```python
from build123d import *

# Parameters (mm, degrees)
F0_R     = 7.5
F1_DEPTH = 2
F2_R     = 4
F3_DEPTH = 2.25
F4_R     = 2.2
F5_DEPTH = 4.251
F6_R     = 0.5


with BuildPart() as f1:
    # F0 (on Front) → F1 (new body)
    with BuildSketch(Plane.XZ):
        Circle(F0_R)
    extrude(amount=F1_DEPTH)

    # F2 (on face) → F3 (join)
    with BuildSketch(Plane.XZ.offset(2)):
        Circle(F2_R)
    extrude(amount=F3_DEPTH)

    # F4 (on face) → F5 (cut, through all)
    with BuildSketch(Plane.XZ.offset(4.25)):
        Circle(F4_R)
    extrude(amount=-F5_DEPTH, mode=Mode.SUBTRACT)

    # F6
    f6_edges = [f1.edges().sort_by_distance(p)[0] for p in [
        (-7.5, 0, 0),
    ]]
    fillet(f6_edges, radius=F6_R)


solid = f1.part
```
Can you work these out from the model? Positions are in its coordinate system, mm. A direction names the side the tool comes from. Give positions to 0.01 mm unless a question says otherwise; leave off trailing zeros. Order: outer loops, then holes, each group sorted by start corner. A loop starts at its lowest first (then second) coordinate and runs counter-clockwise, first axis right, second up. Notation, with made-up numbers: (23, 37) - (60, 37) arc R21 ccw to (60, 62) - close; hole circle Ø9 at (50.5, -8.75). An arc over 180 degrees is marked (long way). Use a Markdown table: item, result. Add a question column.
Q1. On a 3-axis mill with a long thin cutter (end or side, diameter ignored), from which of +Z, -Z, +X, -X, +Y, -Y can I reach the whole of each face in a straight line? I mean faces 4 (the flat face through (-2, 0, 2)), 5 (the flat face through (3, -2, -3)). Say none if no direction works.
Q2. If we section it at B-B on x = 0: Write out the boundary of the cut face in (y, z).
Q3. I'm going to push a flat-ended pin straight in: pin 1 (2 mm diameter, centred on x = -2, y = -2, fed in from -Z). Where does the tip first touch, or does it pass through?
Q4. If we section it at D-D on y = -3.35: Write out the boundary of the cut face in (x, z).
Q5. If we section it at C-C on y = -1.6: Write out the boundary of the cut face in (x, z).
Q6. If we mould it in two halves opening along Z, with no side actions, what happens to faces 1 (the cylindrical face through (-7.493, -1.24, 0.33)), 2 (the cylindrical face through (2.1, -2.15, 0.66)), 3 (the flat face through (2, -4.25, -2))? For each: released by +Z, released by -Z, zero draft, split by the parting line, or undercut.
Q7. Please list where these lines run through material, in increasing order: line 1 along Z through (x, y) = (0, -2.9); line 2 along Y through (x, z) = (-5.5, -2.5); line 3 along X through (y, z) = (-2.8, 1.75).
Q8. If we section it at A-A on z = 0: Write out the boundary of the cut face in (x, y), plus the area to 3 significant figures.
Answers follow:
| question | item | result |
|---|---|---|
| 1 | face 4 | +Z, -Z, +X, -X, +Y |
| 1 | face 5 | -Y |
| 2 | outline | (-4.25, -4) - (-2, -4) - (-2, -7.5) - (-0.5, -7.5) arc R0.5 ccw to (0, -7) - (0, -2.2) - (-4.25, -2.2) - close; (-4.25, 2.2) - (0, 2.2) - (0, 7) arc R0.5 ccw to (-0.5, 7.5) - (-2, 7.5) - (-2, 4) - (-4.25, 4) - close |
| 3 | pin 1 | stops at z = -7.43 |
| 4 | outline | circle Ø8 at (0, 0); hole circle Ø4.4 at (0, 0) |
| 5 | outline | circle Ø15 at (0, 0); hole circle Ø4.4 at (0, 0) |
| 6 | face 1 | split by the parting line |
| 6 | face 2 | undercut |
| 6 | face 3 | zero draft |
| 7 | line 1 | z = -4 to -2.2, 2.2 to 4 |
| 7 | line 2 | y = -2 to 0 |
| 7 | line 3 | x = -3.6 to -1.33, 1.33 to 3.6 |
| 8 | outline | (-7.5, -2) - (-4, -2) - (-4, -4.25) - (-2.2, -4.25) - (-2.2, 0) - (-7, 0) arc R0.5 ccw to (-7.5, -0.5) - close; (2.2, -4.25) - (4, -4.25) - (4, -2) - (7.5, -2) - (7.5, -0.5) arc R0.5 ccw to (7, 0) - (2.2, 0) - close |
| 8 | area | 29.2 mm^2 |
